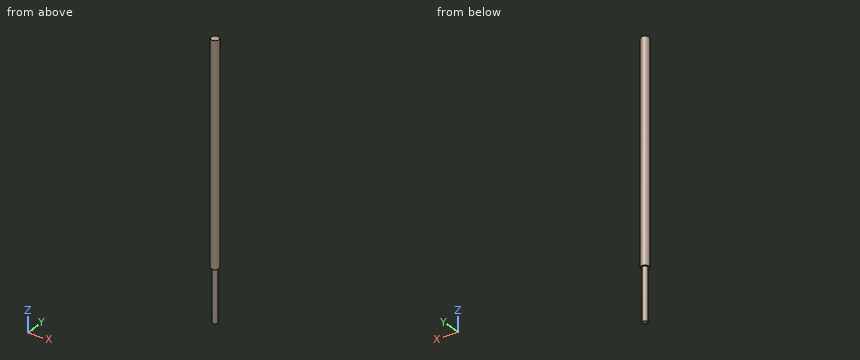
Autodesk Inventor part; units mm, degrees
ref_plane "YZ Plane" through (0, 0, 0) normal (1, 0, 0) x (0, 1, 0)
ref_plane "XZ Plane" through (0, 0, 0) normal (0, 1, 0) x (-1, 0, 0)
ref_plane "XY Plane" through (0, 0, 0) normal (0, 0, 1) x (1, 0, 0)
sketch "Sketch1" plane through (0, 0, 0) normal (0, 0, 1) x (1, 0, 0)
  circle A0 centre (0, 0) radius 25
  dimension "d0" = 50
extrude "Extrusion1" add sketch "Sketch1" along normal blind 10
sketch "Sketch2" plane through (0, 0, 10) normal (0, 0, 1) x (1, 0, 0)
  circle A0 centre (0, 0) radius 6.5
  dimension "d3" = 13
extrude "Extrusion2" add sketch "Sketch2" along normal blind 100
fillet "Fillet1" radius 1 1 edges at (-6.5, 0, 10)
sketch "Sketch4" plane through (0, 0, 0) normal (0, 0, -1) x (-1, 0, 0)
  arc A0 (19.3649, 5) -> (5, 19.3649) centre (0, 0) ccw
  line L0 (2.5, 17.4284) -> (2.5, 9.4868)
  line L1 (9.4868, 2.5) -> (17.4284, 2.5)
  arc A1 (5, 19.3649) -> (2.5, 17.4284) centre (4.5, 17.4284) ccw
  arc A2 (17.4284, 2.5) -> (19.3649, 5) centre (17.4284, 4.5) ccw
  arc A3 (2.5, 8.3666) -> (2.5153, 8.1193) centre (4.5, 8.3666) ccw
  arc A4 (8.1193, 2.5153) -> (8.3666, 2.5) centre (8.3666, 4.5) ccw
  arc A5 (7.6798, 3.6429) -> (3.6429, 7.6798) centre (0, 0) ccw
  arc A6 (2.5, 9.4868) -> (3.6429, 7.6798) centre (4.5, 9.4868) ccw
  arc A7 (7.6798, 3.6429) -> (9.4868, 2.5) centre (9.4868, 4.5) ccw
  point P0 (2.5, 19.8431)
  point P1 (19.8431, 2.5)
  point P2 (2.5, 7.0711)
  point P3 (7.0711, 2.5)
extrude "Extrusion3" cut sketch "Sketch4" against normal blind 10
pattern_circular "Circular Pattern1" count 4 over 360 about axis through (0, 0, 11) along (0, 0, -1) of "Extrusion3"
sketch "Sketch7" plane through (0, 0, 110) normal (0, 0, 1) x (1, 0, 0)
  circle A0 centre (0, 0) radius 7.5
  dimension "d38" = 15
extrude "Extrusion5" add sketch "Sketch7" along normal blind 417
sketch "Sketch8" plane through (0, 0, 527) normal (0, 0, 1) x (1, 0, 0)
  circle A0 centre (0, 0) radius 6.5
  dimension "d41" = 13
extrude "Extrusion6" add sketch "Sketch8" along normal blind 10
sketch "Sketch9" plane through (0, 0, 537) normal (0, 0, 1) x (1, 0, 0)
  circle A0 centre (0, 0) radius 10
  dimension "d44" = 20
extrude "Extrusion7" add sketch "Sketch9" along normal blind 2.5
thread "Thread1"
sketch "Sketch10" plane through (0, 0, 539.5) normal (0, 0, 1) x (1, 0, 0)
  circle A0 centre (0, 0) radius 10
extrude "Extrusion8" cut sketch "Sketch10" against normal blind 12.5
sketch "Sketch11" plane through (0, 0, 0) normal (0, 0, -1) x (-1, 0, 0)
  circle A0 centre (0, 0) radius 25
  circle A1 centre (0, 0) radius 25
extrude "Extrusion9" cut sketch "Sketch11" against normal blind 110
sketch "Sketch12" plane through (0, 0, 110) normal (0, 0, -1) x (-1, 0, 0)
  circle A0 centre (0, 0) radius 5
  dimension "d53" = 10
extrude "Extrusion10" add sketch "Sketch12" along normal blind 100
properties part number "leadscrew_latest" material "Steel, Alloy"
Here's how the part is built. I have some questions about the finished solid (model axes, mm). Coordinates: 2 decimals unless noted, no trailing zeros. Write each loop counter-clockwise with the first axis right and the second up, starting at its lowest first coordinate (ties: lowest second). Pieces come first, ordered by that corner, then holes.
Item 1: I want a section at C-C on z = 170. Write out the boundary of the cut face in (x, y).
Item 2: If I drill on line 1 (Y direction, x = 5.5, z = 241.5); line 2 (X direction, y = -0.5, z = 284.5); line 3 (Z direction, x = -3, y = -6), over which ranges is the centre line in solid material (lowest first)?
Item 3: Will these pins go through, and if not, where does the flat tip stop? pin 1 (1 mm diameter, centred on x = 2, z = 102, fed in from -Y); pin 2 (4 mm diameter, centred on y = -5.5, z = 435.5, fed in from -X); pin 3 (3 mm diameter, centred on x = 2, z = 193.5, fed in from -Y).
Item 4: I want a section at A-A on x = 0. Write out the boundary of the cut face in (y, z), and give its area (4 significant figures).
Findings below:
1. outline: circle Ø15 at (0, 0)
2. line 1: y = -5.1 to 5.1
2. line 2: x = -7.48 to 7.48
2. line 3: z = 110 to 527
3. pin 1: stops at y = -4.77
3. pin 2: stops at x = -6.63
3. pin 3: stops at y = -7.48
4. outline: (-7.5, 110) - (-5, 110) - (-5, 10) - (5, 10) - (5, 110) - (7.5, 110) - (7.5, 527) - (-7.5, 527) - close
4. area: 7,255 mm2
